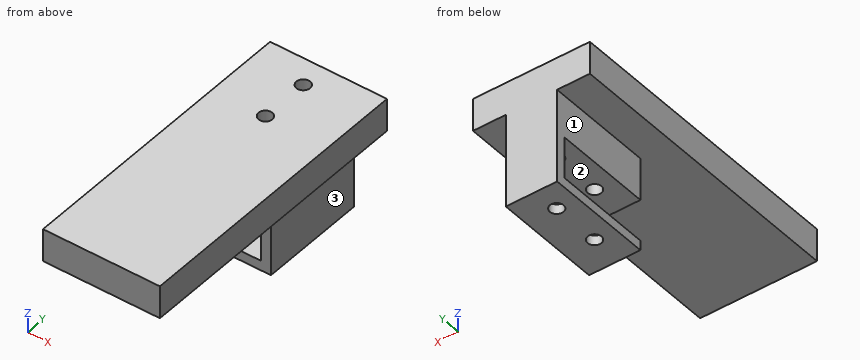
from build123d import *

# Parameters (mm, degrees)
SKETCH3_W             = 18.7
SKETCH3_H             = 18.7
SKETCH3_W_2           = 12.7
SKETCH3_H_2           = 12.7
BOSS_EXTRUDE2_DEPTH   = 30
SKETCH4_W             = 18.7
SKETCH4_H             = 18.7
BOSS_EXTRUDE3_DEPTH   = 3
SKETCH13_W            = 3.048327816
SKETCH13_H            = 18.7
CUT_EXTRUDE1_DEPTH    = 33
SKETCH16_W            = 15.651672184
SKETCH16_H            = 33
BOSS_EXTRUDE6_DEPTH   = 10
SKETCH17_W            = 35.651672184
SKETCH17_H            = 90
BOSS_EXTRUDE7_DEPTH   = 10
M5X0_8_TAPPED_HOLE1_D = 4.2


with BuildPart() as part:
    # Sketch3 → Boss-Extrude2 (new body)
    with BuildSketch(Plane(origin=(0, 0, 0), x_dir=(1, 0, 0), z_dir=(0, 1, 0))):
        with Locations((9.35, 9.35)):
            Rectangle(SKETCH3_W, SKETCH3_H)
        with Locations((9.35, 9.35)):
            Rectangle(SKETCH3_W_2, SKETCH3_H_2, mode=Mode.SUBTRACT)
    extrude(amount=BOSS_EXTRUDE2_DEPTH)

    # Sketch4 → Boss-Extrude3 (add)
    with BuildSketch(Plane(origin=(0, 30, 0), x_dir=(1, 0, 0), z_dir=(0, 1, 0))):
        with Locations((9.35, 9.35)):
            Rectangle(SKETCH4_W, SKETCH4_H)
    extrude(amount=BOSS_EXTRUDE3_DEPTH)

    # Sketch13 → Cut-Extrude1 (cut)
    with BuildSketch(Plane.XZ):
        with Locations((1.524163908, -9.35)):
            Rectangle(SKETCH13_W, SKETCH13_H)
    extrude(amount=-CUT_EXTRUDE1_DEPTH, mode=Mode.SUBTRACT)

    # Sketch16 → Boss-Extrude6 (add)
    with BuildSketch(Plane.XY):
        with Locations((10.874163908, 16.5)):
            Rectangle(SKETCH16_W, SKETCH16_H)
    extrude(amount=BOSS_EXTRUDE6_DEPTH)

    # Sketch17 → Boss-Extrude7 (add)
    with BuildSketch(Plane.XY.offset(10)):
        with Locations((10.874163908, -12)):
            Rectangle(SKETCH17_W, SKETCH17_H)
    extrude(amount=BOSS_EXTRUDE7_DEPTH)

    # M5x0.8 Tapped Hole1 (through all)
    with Locations(Plane(origin=(9.398327816, 24.9, -18.7), x_dir=(-1, 0, 0), z_dir=(0, 0, -1))):
        with Locations((0, 0), (0, -15)):
            Hole(M5X0_8_TAPPED_HOLE1_D / 2)


solid = part.part
CAD build for the part. Positions are in the model's coordinates, mm. Face numbers are marked on the shaded views. A direction names the side the tool comes from. Round coordinates to 2 decimals unless told otherwise and drop trailing zeros. Order: outer loops, then holes, each group sorted by start corner. A loop starts at its lowest first (then second) coordinate and runs counter-clockwise, first axis right, second up. Notation, with made-up numbers: (12.5, 53) - (32.5, 53) arc R30 ccw to (32.5, 91) - close; hole circle Ø3 at (1.5, 75.25). An arc over 180 degrees is marked (long way). Return JSON: item names as keys, results as strings.
(1) Pin check, flat tips, straight feed: pin 1 Ø8.5 at (y, z) = (24, 1.5) entering from -X; pin 2 Ø2 at (y, z) = (-2, 7.5) entering from +X; pin 3 Ø12.5 at (x, z) = (11.5, -5.5) entering from -Y; pin 4 Ø4 at (x, y) = (-1, 3) entering from -Z. Stop position of each tip, or through.
Answer key:
{"pin 1": "stops at x = 3.05", "pin 2": "passes through", "pin 3": "stops at y = 0", "pin 4": "stops at z = 10"}
(2) Cut at B-B (z = 6.5). Give the cut face in (x, y).
Answer key:
{"outline": "(3.05, 0) - (18.7, 0) - (18.7, 33) - (3.05, 33) - close; hole circle Ø4.2 at (9.4, 9.9); hole circle Ø4.2 at (9.4, 24.9)"}
(3) Tool access for the marked faces 1, 2 and 3: list every direction of +Z, -Z, +X, -X, +Y, -Y with a clear straight run to the whole face (end or side of a thin tool).
Answer key:
{"face 1": "-Z, -X, +Y, -Y", "face 2": "-X, -Y", "face 3": "-Z, +X, +Y, -Y"}
(4) Wall check: probe 1 along Z at (x, y) = (11, -33); probe 2 along X at (y, z) = (25, -16); probe 3 along X at (y, z) = (19, 3). Give the ranges that are in metal, low to high. Write a range as from..to.
Answer key:
{"probe 1": "z = 10..20", "probe 2": "x = 3.05..7.3, 11.5..18.7", "probe 3": "x = 3.05..18.7"}
(5) Cut at A-A (y = 24.9). Give the cut face in (x, z).
Answer key:
{"outline": "(-6.95, 10) - (3.05, 10) - (3.05, -3) - (7.3, -3) - (7.3, 20) - (-6.95, 20) - close; (3.05, -18.7) - (7.3, -18.7) - (7.3, -15.7) - (3.05, -15.7) - close; (11.5, -18.7) - (18.7, -18.7) - (18.7, 10) - (28.7, 10) - (28.7, 20) - (11.5, 20) - (11.5, -3) - (15.7, -3) - (15.7, -15.7) - (11.5, -15.7) - close"}
(6) Cut at C-C (x = 9). Give the cut face in (y, z), then the cut area to 3 significant figures.
Answer key:
{"outline": "(-57, 10) - (0, 10) - (0, -3) - (7.84, -3) - (7.84, 20) - (-57, 20) - close; (0, -18.7) - (7.84, -18.7) - (7.84, -15.7) - (0, -15.7) - close; (11.96, -18.7) - (22.84, -18.7) - (22.84, -15.7) - (11.96, -15.7) - close; (11.96, -3) - (22.84, -3) - (22.84, 20) - (11.96, 20) - close; (26.96, -18.7) - (33, -18.7) - (33, 20) - (26.96, 20) - (26.96, -3) - (30, -3) - (30, -15.7) - (26.96, -15.7) - close", "area": "1,250 mm^2"}
(7) Cut at D-D (y = -30). Give the cut face in (x, z), then the cut area to 3 significant figures.
Answer key:
{"outline": "(-6.95, 10) - (28.7, 10) - (28.7, 20) - (-6.95, 20) - close", "area": "357 mm^2"}
